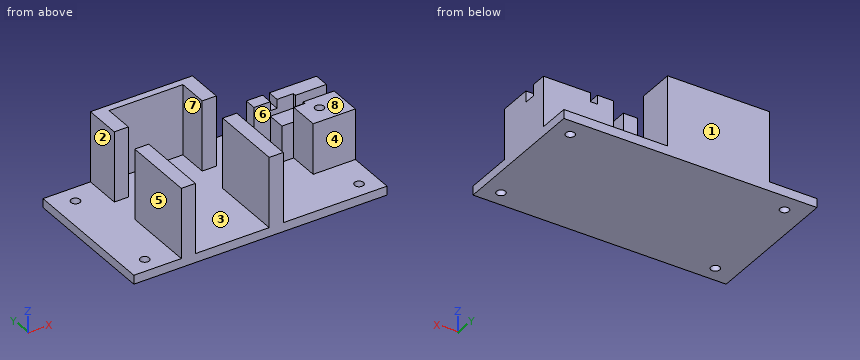
```python
from build123d import *

# Parameters (mm, degrees)
SKETCH1_W            = 180
SKETCH1_H            = 100
BOSS_EXTRUDE1_DEPTH  = 6.35
SKETCH2_W            = 26.25
SKETCH2_H            = 5
BOSS_EXTRUDE3_DEPTH  = 50
SKETCH3_W            = 30
SKETCH3_H            = 30
BOSS_EXTRUDE4_DEPTH  = 25.65
BOSS_EXTRUDE5_DEPTH  = 10.35
SKETCH5_W            = 22
SKETCH5_H            = 8.5
BOSS_EXTRUDE6_DEPTH  = 2.35
SKETCH6_W            = 20
SKETCH6_H            = 8.5
BOSS_EXTRUDE7_DEPTH  = 29.625
SKETCH8_W            = 3.625
SKETCH8_H            = 8.5
SKETCH8_W_2          = 11.625
BOSS_EXTRUDE8_DEPTH  = 6.375
SKETCH9_W            = 8.375
SKETCH9_H            = 12.8
BOSS_EXTRUDE9_DEPTH  = 25.65
SKETCH10_R           = 3.175
CUT_EXTRUDE1_DEPTH   = 6.35
SKETCH11_W           = 30
SKETCH11_H           = 12.7
BOSS_EXTRUDE10_DEPTH = 36
SKETCH12_R           = 3.175
CUT_EXTRUDE2_DEPTH   = 10


with BuildPart() as part:
    # Sketch1 → Boss-Extrude1 (new body)
    with BuildSketch(Plane.XY):
        with Locations((90, 50)):
            Rectangle(SKETCH1_W, SKETCH1_H)
    extrude(amount=BOSS_EXTRUDE1_DEPTH)

    # Sketch2 → Boss-Extrude3 (add)
    with BuildSketch(Plane.XY.offset(6.35)):
        Polygon((43.75, 95), (43.75, 100), (33.75, 100), (33.75, 73.75), (43.75, 73.75), align=None)
        with Locations((56.875, 97.5)):
            Rectangle(SKETCH2_W, SKETCH2_H)
        with Locations((83.125, 97.5)):
            Rectangle(SKETCH2_W, SKETCH2_H)
        Polygon((106.25, 100), (96.25, 100), (96.25, 95), (96.25, 73.75), (106.25, 73.75), align=None)
        Polygon((33.75, 0), (43.75, 0), (43.75, 5), (43.75, 51.25), (33.75, 51.25), align=None)
        Polygon((96.25, 5), (96.25, 0), (106.25, 0), (106.25, 51.25), (96.25, 51.25), align=None)
    extrude(amount=BOSS_EXTRUDE3_DEPTH)

    # Sketch3 → Boss-Extrude4 (add)
    with BuildSketch(Plane.XY.offset(6.35)):
        with Locations((165, 62.5)):
            Rectangle(SKETCH3_W, SKETCH3_H)
    extrude(amount=BOSS_EXTRUDE4_DEPTH)

    # Sketch4 → Boss-Extrude5 (add)
    with BuildSketch(Plane.XY.offset(32)):
        Polygon((150, 77.5), (150, 69), (158, 69), (158, 66.75), (180, 66.75), (180, 77.5), align=None)
        Polygon((158, 56.2), (150, 56.2), (150, 47.5), (180, 47.5), (180, 58.25), (158, 58.25), align=None)
    extrude(amount=BOSS_EXTRUDE5_DEPTH)

    # Sketch5 → Boss-Extrude6 (add)
    with BuildSketch(Plane.XY.offset(32)):
        with Locations((169, 62.5)):
            Rectangle(SKETCH5_W, SKETCH5_H)
    extrude(amount=BOSS_EXTRUDE6_DEPTH)

    # Sketch6 → Boss-Extrude7 (add)
    with BuildSketch(Plane.XY.offset(6.35)):
        with Locations((140, 73.25)):
            Rectangle(SKETCH6_W, SKETCH6_H)
    extrude(amount=BOSS_EXTRUDE7_DEPTH)

    # Sketch8 → Boss-Extrude8 (add)
    with BuildSketch(Plane.XY.offset(35.975)):
        with Locations((148.1875, 73.25)):
            Rectangle(SKETCH8_W, SKETCH8_H)
        with Locations((135.8125, 73.25)):
            Rectangle(SKETCH8_W_2, SKETCH8_H)
    extrude(amount=BOSS_EXTRUDE8_DEPTH)

    # Sketch9 → Boss-Extrude9 (add)
    with BuildSketch(Plane.XY.offset(6.35)):
        with Locations((145.8125, 62.6)):
            Rectangle(SKETCH9_W, SKETCH9_H)
    extrude(amount=BOSS_EXTRUDE9_DEPTH)

    # Sketch10 → Cut-Extrude1 (cut)
    with BuildSketch(Plane.XY.offset(6.35)):
        with Locations((14.9, 87.3)):
            Circle(SKETCH10_R)
        with Locations((167.3, 87.3)):
            Circle(SKETCH10_R)
        with Locations((167.3, 11.1)):
            Circle(SKETCH10_R)
        with Locations((14.9, 11.1)):
            Circle(SKETCH10_R)
    extrude(amount=-CUT_EXTRUDE1_DEPTH, mode=Mode.SUBTRACT)

    # Sketch11 → Boss-Extrude10 (add)
    with BuildSketch(Plane.XY.offset(6.35)):
        with Locations((165, 41.15)):
            Rectangle(SKETCH11_W, SKETCH11_H)
    extrude(amount=BOSS_EXTRUDE10_DEPTH)

    # Sketch12 → Cut-Extrude2 (cut)
    with BuildSketch(Plane.XY.offset(42.35)):
        with Locations((162.7, 47.5)):
            Circle(SKETCH12_R)
    extrude(amount=-CUT_EXTRUDE2_DEPTH, mode=Mode.SUBTRACT)


solid = part.part
```
The model under review builds one solid part; all positions refer to its coordinate system, in mm. Face numbers are marked on the shaded views. A direction names the side the tool comes from. Round coordinates to 2 decimals unless told otherwise and drop trailing zeros. Write each loop counter-clockwise with the first axis right and the second up, starting at its lowest first coordinate (ties: lowest second). Pieces come first, ordered by that corner, then holes.
(1) We need section B-B on y = 87.3. Give the boundary of the cut face in (x, z) (3 decimals).
(2) Mouldability with a two-part tool opening along X and no side actions: class the marked faces 1, 2 and 3 as +X half, -X half, draft (parallel to the pull), parting line (faces both ways), or undercut.
(3) We need section C-C on x = 14.9. Give the boundary of the cut face in (y, z) (3 decimals).
(4) We need section D-D on z = 51. Give the boundary of the cut face in (x, y), and give its area (3 significant figures).
(5) We need section A-A on z = 13. Give the boundary of the cut face in (x, y) (3 decimals), and give its area (3 significant figures).
(6) Machinability: for the marked faces 4, 5, 6, 7 and 8, which of the approach directions +Z, -Z, +X, -X, +Y, -Y give a long, thin tool a straight path to every point of the face, cutting with its end or side? Answer none if there is none.
(7) Insertion check: pin 1 (5 mm diameter, centred on x = 144, y = 75, fed in from +Z); pin 2 (4 mm diameter, centred on x = 152, y = 63, fed in from +Z); pin 3 (1 mm diameter, centred on y = 89.5, z = 42, fed in from +X). Each pin has a flat end and moves straight along its axis. Give the tip position at first contact, or say it passes through.
(8) Wall thickness on L1, parallel to Y at x = 167.3, z = 2.5 (3 decimals); L2, parallel to Y at x = 162.7, z = 39.75 (3 decimals); L3, parallel to X at y = 47, z = 38: over which ranges is each line inside the solid? List them lowest first.
Findings below:
1. outline: (0, 0) - (11.725, 0) - (11.725, 6.35) - (0, 6.35) - close; (18.075, 0) - (164.125, 0) - (164.125, 6.35) - (106.25, 6.35) - (106.25, 56.35) - (96.25, 56.35) - (96.25, 6.35) - (43.75, 6.35) - (43.75, 56.35) - (33.75, 56.35) - (33.75, 6.35) - (18.075, 6.35) - close; (170.475, 0) - (180, 0) - (180, 6.35) - (170.475, 6.35) - close
2. face 1: draft
2. face 2: -X half
2. face 3: undercut
3. outline: (0, 0) - (7.925, 0) - (7.925, 6.35) - (0, 6.35) - close; (14.275, 0) - (84.125, 0) - (84.125, 6.35) - (14.275, 6.35) - close; (90.475, 0) - (100, 0) - (100, 6.35) - (90.475, 6.35) - close
4. outline: (33.75, 0) - (43.75, 0) - (43.75, 51.25) - (33.75, 51.25) - close; (33.75, 73.75) - (43.75, 73.75) - (43.75, 95) - (96.25, 95) - (96.25, 73.75) - (106.25, 73.75) - (106.25, 100) - (33.75, 100) - close; (96.25, 0) - (106.25, 0) - (106.25, 51.25) - (96.25, 51.25) - close
4. area: 1,810 mm2
5. outline: (33.75, 0) - (43.75, 0) - (43.75, 51.25) - (33.75, 51.25) - close; (33.75, 73.75) - (43.75, 73.75) - (43.75, 95) - (96.25, 95) - (96.25, 73.75) - (106.25, 73.75) - (106.25, 100) - (33.75, 100) - close; (96.25, 0) - (106.25, 0) - (106.25, 51.25) - (96.25, 51.25) - close; (130, 69) - (141.625, 69) - (141.625, 56.2) - (150, 56.2) - (150, 34.8) - (180, 34.8) - (180, 77.5) - (130, 77.5) - close
5. area: 3,370 mm2
6. face 4: +Z, +X, -Y
6. face 5: +Z, -X, +Y, -Y
6. face 6: +Z, -X
6. face 7: +Z, -Y
6. face 8: +Z, +X, +Y, -Y
7. pin 1: stops at z = 42.35
7. pin 2: stops at z = 32
7. pin 3: stops at x = 106.25
8. L1: y = 0 to 7.925, 14.275 to 84.125, 90.475 to 100
8. L2: y = 34.8 to 44.325, 50.675 to 58.25, 66.75 to 77.5
8. L3: x = 33.75 to 43.75, 96.25 to 106.25, 150 to 159.56, 165.84 to 180
